Input: part model. Units: mm. Frame: model coordinates. Round coordinates to 2 decimals unless told otherwise and drop trailing zeros. Loops run counter-clockwise (first coordinate to the right, second up) from the corner with the lowest first, then second, coordinate; pieces in that order, holes last. Notation, with made-up numbers: (62.5, 42) -> (120.5, 42) arc R21 ccw to (120.5, 51) -> close; hole circle Ø3 at (77.25, -29). An arc over 180 degrees is marked (long way). One line per question, with ' | ' between items. Start each with the question number.
Q1. Cut plane A-A on x = 1.48. Return loops of the section in (y, z) (3 decimals), and give its area (3 significant figures).
Q2. Material intervals for L1, parallel to Z at x = 1, y = 57; L2, parallel to X at y = 60, z = 26; L3, parallel to X at y = 58.5, z = 7.5, sorted ascending.
Q3. Contact query for flat-ended pins moving along their axis: P1, Ø7, axis at x = -22.52, z = 26, coming from the +Y side (3 decimals); P2, Ø2, axis at x = 8, y = 26, coming from the -Z side. Output: stop coordinate, or through.
Q4. Cut plane C-C on z = 9. Return loops of the section in (x, y) (3 decimals).
Q5. Cut plane B-B on y = 47.5. Return loops of the section in (x, z), and give its area (3 significant figures).
from build123d import *

# Parameters (mm, degrees)
SKETCH2_R           = 3.55
BOSS_EXTRUDE1_DEPTH = 35
SKETCH3_R           = 2.25
CUT_EXTRUDE1_DEPTH  = 110.173579221
SKETCH5_R           = 4
CUT_EXTRUDE3_DEPTH  = 10


with BuildPart() as part:
    # Sketch2 → Boss-Extrude1 (new body)
    with BuildSketch(Plane.XY):
        Polygon((-90.52, 14.235), (-90.52, 64.235), (-25.52, 64.235), (4.48, 64.235), (69.48, 64.235), (69.48, 14.235), align=None)
        with Locations((-60.52, 49.235)):
            Circle(SKETCH2_R, mode=Mode.SUBTRACT)
        with Locations((39.48, 49.235)):
            Circle(SKETCH2_R, mode=Mode.SUBTRACT)
    extrude(amount=BOSS_EXTRUDE1_DEPTH)

    # Sketch3 → Cut-Extrude1 (cut, through all)
    with BuildSketch(Plane.XZ.offset(-14.235)):
        with Locations((-22.52, 26)):
            Circle(SKETCH3_R)
        with Locations((1.48, 26)):
            Circle(SKETCH3_R)
        with Locations((-22.52, 9)):
            Circle(SKETCH3_R)
        with Locations((1.48, 9)):
            Circle(SKETCH3_R)
    extrude(amount=-CUT_EXTRUDE1_DEPTH, mode=Mode.SUBTRACT)

    # Sketch5 → Cut-Extrude3 (cut)
    with BuildSketch(Plane(origin=(0, 64.235, 0), x_dir=(1, 0, 0), z_dir=(0, 1, 0))):
        with Locations(Location((-22.52, -9, 0), (0, 0, 270))):
            Circle(SKETCH5_R)
        with Locations(Location((-22.52, -26, 0), (0, 0, 270))):
            Circle(SKETCH5_R)
        with Locations(Location((1.48, -26, 0), (0, 0, 270))):
            Circle(SKETCH5_R)
        with Locations(Location((1.48, -9, 0), (0, 0, 270))):
            Circle(SKETCH5_R)
    extrude(amount=-CUT_EXTRUDE3_DEPTH, mode=Mode.SUBTRACT)


solid = part.part
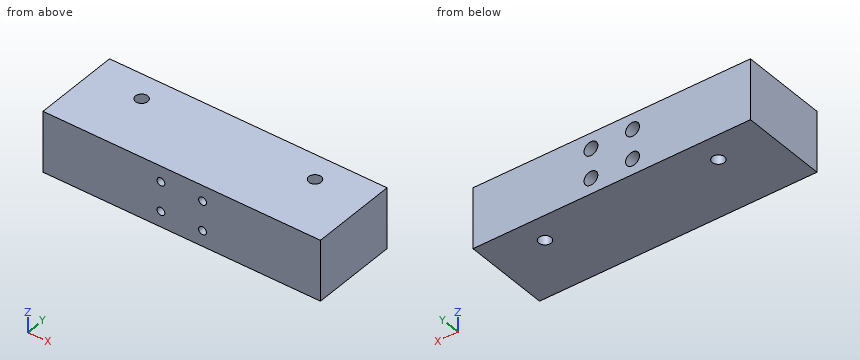
Results:
1) outline: (14.235, 0) -> (64.235, 0) -> (64.235, 5) -> (54.235, 5) -> (54.235, 6.75) -> (14.235, 6.75) -> close; (14.235, 11.25) -> (54.235, 11.25) -> (54.235, 13) -> (64.235, 13) -> (64.235, 22) -> (54.235, 22) -> (54.235, 23.75) -> (14.235, 23.75) -> close; (14.235, 28.25) -> (54.235, 28.25) -> (54.235, 30) -> (64.235, 30) -> (64.235, 35) -> (14.235, 35) -> close | area: 1,230 mm^2
2) L1: 0 to 5.03, 12.97 to 22.03, 29.97 to 35 | L2: -90.52 to -26.52, -18.52 to -2.52, 5.48 to 69.48 | L3: -90.52 to -26.23, -18.81 to -2.23, 5.19 to 69.48
3) P1: y = 54.235 | P2: z = 0
4) outline: (-90.52, 14.235) -> (-24.77, 14.235) -> (-24.77, 54.235) -> (-26.52, 54.235) -> (-26.52, 64.235) -> (-90.52, 64.235) -> close; (-20.27, 14.235) -> (-0.77, 14.235) -> (-0.77, 54.235) -> (-2.52, 54.235) -> (-2.52, 64.235) -> (-18.52, 64.235) -> (-18.52, 54.235) -> (-20.27, 54.235) -> close; (3.73, 14.235) -> (69.48, 14.235) -> (69.48, 64.235) -> (5.48, 64.235) -> (5.48, 54.235) -> (3.73, 54.235) -> close; hole circle Ø7.1 at (-60.52, 49.235); hole circle Ø7.1 at (39.48, 49.235)
5) outline: (-90.52, 0) -> (-63.62, 0) -> (-63.62, 35) -> (-90.52, 35) -> close; (-57.42, 0) -> (36.38, 0) -> (36.38, 35) -> (-57.42, 35) -> close; (42.58, 0) -> (69.48, 0) -> (69.48, 35) -> (42.58, 35) -> close; hole circle Ø4.5 at (-22.52, 9); hole circle Ø4.5 at (-22.52, 26); hole circle Ø4.5 at (1.48, 9); hole circle Ø4.5 at (1.48, 26) | area: 5,100 mm^2
